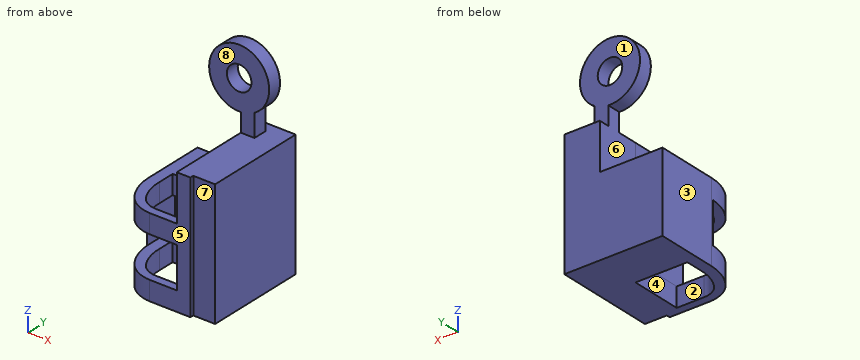
from build123d import *

# Parameters (mm, degrees)
BOSS_EXTRUDE1_DEPTH     = 46
SKETCH3_W               = 23
SKETCH3_H               = 15
CUT_EXTRUDE2_DEPTH      = 28
CUT_EXTRUDE6_DEPTH      = 40
CUT_EXTRUDE6_DEPTH_BACK = 30
SKETCH10_W              = 22.999996183
SKETCH10_H              = 16.921181255
SKETCH7_R               = 11
SKETCH7_R_2             = 4.5
BOSS_EXTRUDE2_DEPTH     = 5
BOSS_EXTRUDE3_DEPTH     = 5


with BuildPart() as part:
    # Sketch1 → Boss-Extrude1 (new body)
    with BuildSketch(Plane.XY):
        with BuildLine():
            Line((-22.718454064, 23.966100395), (13.281542119, 23.93479699))
            Line((13.281542119, 23.93479699), (13.281542119, -13.210798183))
            Line((13.281542119, -13.210798183), (5.281545459, -13.210798183))
            Line((5.281545459, -13.210798183), (5.281545459, -14.529188453))
            Line((5.281545459, -14.529188453), (-9.718454064, -14.529188453))
            ThreePointArc((-9.718454064, -14.529188453), (-14.925713646, -13.200176165), (-19.056981743, -9.762960731))
            ThreePointArc((-19.056981743, -9.762960731), (-21.779979177, -4.437922335), (-22.718454064, 1.468854607))
            Line((-22.718454064, 1.468854607), (-22.718454064, 23.966100395))
        make_face()
        with BuildLine():
            Line((-18.718455971, 7.468114556), (0.281544029, 7.468114556))
            Line((0.281544029, 7.468114556), (0.281544029, -11.529558479))
            Line((0.281544029, -11.529558479), (-9.718454064, -11.529558479))
            ThreePointArc((-9.718454064, -11.529558479), (-13.398330557, -10.623193541), (-16.168405236, -8.036752998))
            ThreePointArc((-16.168405236, -8.036752998), (-18.168441603, -3.478446477), (-18.718455971, 1.468854607))
            Line((-18.718455971, 1.468854607), (-18.718455971, 7.468114556))
        make_face(mode=Mode.SUBTRACT)
    extrude(amount=BOSS_EXTRUDE1_DEPTH)

    # Sketch3 → Cut-Extrude2 (cut)
    with BuildSketch(Plane.XZ.offset(14.529188453)):
        with Locations((-11.2030368, 14.578818745)):
            Rectangle(SKETCH3_W, SKETCH3_H)
    extrude(amount=-CUT_EXTRUDE2_DEPTH, mode=Mode.SUBTRACT)

    # Sketch10 → Cut-Extrude6 (cut, two sides: drawn at the far end of the back side and taken through both)
    with BuildSketch(Plane(origin=(0, 7.468114556, 0), x_dir=(-1, 0, 0), z_dir=(0, -1, 0)).offset(-CUT_EXTRUDE6_DEPTH_BACK)):
        with Locations((11.218455973, -37.539409373)):
            Rectangle(SKETCH10_W, SKETCH10_H)
    extrude(amount=CUT_EXTRUDE6_DEPTH + CUT_EXTRUDE6_DEPTH_BACK, mode=Mode.SUBTRACT)



with BuildPart() as body_2:
    # Sketch7 → Boss-Extrude2 (new body)
    with BuildSketch(Plane(origin=(0, 20, 0), x_dir=(1, 0, 0), z_dir=(0, 1, 0))):
        with Locations(Location((-0.321447284, -63.773621976, 0), (0, 0, 270))):
            Circle(SKETCH7_R)
        with Locations(Location((-0.321447284, -63.773621976, 0), (0, 0, 270))):
            Circle(SKETCH7_R_2, mode=Mode.SUBTRACT)
    extrude(amount=-BOSS_EXTRUDE2_DEPTH)


with BuildPart() as part_1:
    add(part.part)

    add(body_2.part)  # Boss-Extrude3 merges body 2
    # Sketch12 → Boss-Extrude3 (add)
    with BuildSketch(Plane(origin=(0, 20, 0), x_dir=(1, 0, 0), z_dir=(0, 1, 0))):
        with BuildLine():
            Line((0.281542119, -46), (0.281542119, -52.790161511))
            ThreePointArc((0.281542119, -52.790161511), (2.872949751, -53.247662277), (5.281545459, -54.307552448))
            Line((5.281545459, -54.307552448), (5.281545459, -46))
            Line((5.281545459, -46), (0.281542119, -46))
        make_face()
    extrude(amount=-BOSS_EXTRUDE3_DEPTH)


solid = part_1.part
Model file for the job. Use its own axes, mm. Face numbers are marked on the shaded views. A direction names the side the tool comes from. Give positions to 0.01 mm unless a question says otherwise; leave off trailing zeros. Order: outer loops, then holes, each group sorted by start corner. A loop starts at its lowest first (then second) coordinate and runs counter-clockwise, first axis right, second up. Notation, with made-up numbers: (89, -12.5) -> (117, -12.5) arc R22 cw to (117, 3.5) -> close; hole circle Ø9 at (-25, 57). An arc over 180 degrees is marked (long way). Use CSV: the item, a comma, the result in double quotes.
1. 3-axis set-ups, long thin cutter, end or side, ignore diameter. For the marked faces 5, 6, 7 and 8: which of +Z, -Z, +X, -X, +Y, -Y reach the whole face in a straight line?
Outcome:
face 5,"+Z, -Z, +X, -X, -Y"
face 6,"-X, +Y, -Y"
face 7,"+Z, -Z, +X, -Y"
face 8,"+Z, +X, -X, -Y"
2. Drill centre lines: line 1 along Y through (x, z) = (-9, 24.5); line 2 along Z through (x, y) = (2.5, 20.5). Where is each one in solid material? Low to high. Write a range as from..to.
Outcome:
line 1,"-14.53..-11.53, 7.47..23.95"
line 2,"0..46"
3. Drop flat-ended pins along their axis: pin 1 (11.5 mm diameter, centred on x = -15, y = 3, fed in from +Z); pin 2 (3.5 mm diameter, centred on x = -7, z = 4.5, fed in from +Y); pin 3 (6 mm diameter, centred on x = 6, y = 6.5, fed in from +Z). Give the stop position or say it passes through.
Outcome:
pin 1,"z = 29.08"
pin 2,"y = 23.95"
pin 3,"z = 46"
4. Mould opens along Y. For the marked faces 1, 2, 3 and 4 say: +Y half, -Y half, draft (parallel to the pull), parting line (faces both ways), or undercut.
Outcome:
face 1,"+Y half"
face 2,"undercut"
face 3,"draft"
face 4,"undercut"
5. Band-saw the part on D-D, the plane y = -6. Count the separate pieces of the cut face and the enclosed holes in it, then the cut area to 3 significant figures.
Outcome:
separate pieces,"3"
enclosed holes,"0"
area,"653 mm²"
6. Band-saw the part on B-B, the plane x = 2. Give the cut face in (y, z).
Outcome:
outline,"(-14.53, 0) -> (23.94, 0) -> (23.94, 46) -> (20, 46) -> (20, 59.92) -> (15, 59.92) -> (15, 46) -> (-14.53, 46) -> close; (15, 67.63) -> (20, 67.63) -> (20, 74.53) -> (15, 74.53) -> close"
7. Band-saw the part on C-C, the plane z = 14. Give the cut face in (x, y).
Outcome:
outline,"(-22.72, 1.47) arc R19.06 ccw to (-22.7, 0.7) -> (-22.7, 13.47) -> (0.3, 13.47) -> (0.3, -14.53) -> (5.28, -14.53) -> (5.28, -13.21) -> (13.28, -13.21) -> (13.28, 23.93) -> (-22.72, 23.97) -> close"
